from build123d import *

# Parameters (mm, degrees)
F4_D           = 6.8
F4_DEPTH       = 5
F4_CSINK_D     = 8
F4_CSINK_ANGLE = 90


with BuildPart() as f2:
    # F2: sweep along a path in F1
    with BuildLine(Plane.YZ) as f2_path:
        Line((0, 0), (-150, 0))
    # F0 (on Front) → F2 (sweep)
    with BuildSketch(Plane.XZ):
        with BuildLine():
            Line((30, 0), (0, 0))
            Line((0, 0), (0, -30))
            Line((0, -30), (1.5, -30))
            ThreePointArc((1.5, -30), (2.56066, -29.56066), (3, -28.5))
            Line((3, -28.5), (3, -4))
            ThreePointArc((3, -4), (3.292893, -3.292893), (4, -3))
            Line((4, -3), (28.5, -3))
            ThreePointArc((28.5, -3), (29.56066, -2.56066), (30, -1.5))
            Line((30, -1.5), (30, 0))
        make_face()
    sweep(path=f2_path.line)

    # F4
    with Locations(Plane.XY):
        with Locations((15, -125), (15, -25)):
            CounterSinkHole(F4_D / 2, F4_CSINK_D / 2, depth=F4_DEPTH, counter_sink_angle=F4_CSINK_ANGLE)


solid = f2.part
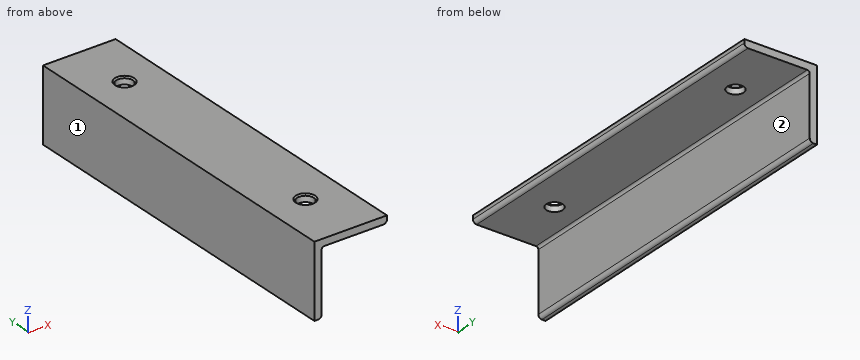
Can you work these out from the model? Positions are in its coordinate system, mm. Face numbers are marked on the shaded views. A direction names the side the tool comes from. Give positions to 0.01 mm unless a question says otherwise; leave off trailing zeros. Loops run counter-clockwise (first coordinate to the right, second up) from the corner with the lowest first, then second, coordinate; pieces in that order, holes last. Notation, with made-up numbers: M 27,-39 L 64,-39 A15 ccw 64,-17 Z; hole C 72.25,22.25 d4. An arc over 180 degrees is marked long. One line per item, written item: value. Start each with the question number.
1) If we section it at B-B, the plane x = 15: Write out the boundary of the cut face in (y, z), and give its area (3 significant figures).
2) If I drill on line 1 (Y direction, x = 15, z = -1.7); line 2 (X direction, y = -125, z = -1.6); line 3 (Z direction, x = 12, y = -16.5), over which ranges is the centre line in solid material (lowest first)? Write a range as [from, to].
3) I'm going to push flat-ended pins straight in: pin 1 (8 mm diameter, centred on x = 15, y = -25, fed in from -Z); pin 2 (10 mm diameter, centred on y = -86, z = -26.5, fed in from +X). Where does each tip first touch, or does it pass through?
4) If we section it at C-C, the plane y = -131: Write out the boundary of the cut face in (x, z).
5) If we section it at D-D, the plane x = 21: Write out the boundary of the cut face in (y, z).
6) If we section it at A-A, the plane y = -25: Write out the boundary of the cut face in (x, z), and give its area (3 significant figures).
7) On a 3-axis mill with a long thin cutter (end or side, diameter ignored), from which of +Z, -Z, +X, -X, +Y, -Y can I reach the whole of each face in a straight line? I mean the marked faces 1 and 2. Say none if no direction works.
Completed:
1. outline: M -150,-3 L -128.4,-3 L -128.4,-0.6 L -129,0 L -150,0 Z; M -121.6,-3 L -28.4,-3 L -28.4,-0.6 L -29,0 L -121,0 L -121.6,-0.6 Z; M -21.6,-3 L 0,-3 L 0,0 L -21,0 L -21.6,-0.6 Z
1. area: 408 mm^2
2. line 1: y = [-150, -128.4], [-121.6, -28.4], [-21.6, 0]
2. line 2: x = [0, 11.6], [18.4, 30]
2. line 3: z = [-3, 0]
3. pin 1: stops at z = -3
3. pin 2: stops at x = 3
4. outline: M 0,-30 L 1.5,-30 A1.5 ccw 3,-28.5 L 3,-4 A1 cw 4,-3 L 28.5,-3 A1.5 ccw 30,-1.5 L 30,0 L 0,0 Z
5. outline: M -150,-3 L 0,-3 L 0,0 L -150,0 Z
6. outline: M 0,-30 L 1.5,-30 A1.5 ccw 3,-28.5 L 3,-4 A1 cw 4,-3 L 11.6,-3 L 11.6,-0.6 L 11,0 L 0,0 Z; M 18.4,-3 L 28.5,-3 A1.5 ccw 30,-1.5 L 30,0 L 19,0 L 18.4,-0.6 Z
6. area: 149 mm^2
7. face 1: +Z, -Z, -X, +Y, -Y
7. face 2: -Z, +X, +Y, -Y
